from build123d import *

# Parameters (mm, degrees)
SKETCH1_W           = 304.8
SKETCH1_H           = 203.2
BOSS_EXTRUDE1_DEPTH = 228.6
SKETCH2_R           = 101.6
SKETCH2_R_2         = 76.2
BOSS_EXTRUDE2_DEPTH = 50.8
SKETCH3_R           = 38.1
CUT_EXTRUDE1_DEPTH  = 38.1
SKETCH4_W           = 203.2
SKETCH4_H           = 203.2
CUT_EXTRUDE2_DEPTH  = 190.5
SKETCH5_R           = 40.64
CUT_EXTRUDE3_DEPTH  = 304.8
FILLET1_R           = 101.6
CHAMFER1_SIZE       = 38.1


with BuildPart() as part:
    # Sketch1 → Boss-Extrude1 (new body)
    with BuildSketch(Plane(origin=(0, 0, 0), x_dir=(1, 0, 0), z_dir=(0, 1, 0))):
        Rectangle(SKETCH1_W, SKETCH1_H)
    extrude(amount=BOSS_EXTRUDE1_DEPTH)

    # Sketch2 → Boss-Extrude2 (add)
    with BuildSketch(Plane(origin=(0, 228.6, 0), x_dir=(1, 0, 0), z_dir=(0, 1, 0))):
        with Locations(Location((0, 0, 0), (0, 0, 270))):
            Circle(SKETCH2_R)
        with Locations(Location((0, 0, 0), (0, 0, 270))):
            Circle(SKETCH2_R_2, mode=Mode.SUBTRACT)
    extrude(amount=BOSS_EXTRUDE2_DEPTH)

    # Sketch3 → Cut-Extrude1 (cut)
    with BuildSketch(Plane(origin=(0, 228.6, 0), x_dir=(1, 0, 0), z_dir=(0, 1, 0))):
        with Locations(Location((0, 0, 0), (0, 0, 270))):
            Circle(SKETCH3_R)
    extrude(amount=-CUT_EXTRUDE1_DEPTH, mode=Mode.SUBTRACT)

    # Sketch4 → Cut-Extrude2 (cut)
    with BuildSketch(Plane.XZ):
        Rectangle(SKETCH4_W, SKETCH4_H)
    extrude(amount=-CUT_EXTRUDE2_DEPTH, mode=Mode.SUBTRACT)

    # Sketch5 → Cut-Extrude3 (cut)
    with BuildSketch(Plane(origin=(152.4, 0, 0), x_dir=(0, 0, -1), z_dir=(1, 0, 0))):
        with Locations((0, 101.6)):
            Circle(SKETCH5_R)
    extrude(amount=-CUT_EXTRUDE3_DEPTH, mode=Mode.SUBTRACT)

    # Fillet1
    fillet1_edges = [part.edges().sort_by_distance(p)[0] for p in [
        (127, 0, -101.6),
        (127, 0, 101.6),
        (-127, 0, -101.6),
        (-127, 0, 101.6),
    ]]
    fillet(fillet1_edges, radius=FILLET1_R - 0.0001)  # a hair under: the kernel refuses the full size

    # Chamfer1
    chamfer1_edges = [part.edges().sort_by_distance(p)[0] for p in [
        (0, 228.6, -38.1),
    ]]
    chamfer(chamfer1_edges, length=CHAMFER1_SIZE - 0.0001)  # a hair under: the kernel refuses the full size


solid = part.part
Model file for the job. Use its own axes, mm. A direction names the side the tool comes from. Coordinates: 2 decimals unless noted, no trailing zeros. Write each loop counter-clockwise with the first axis right and the second up, starting at its lowest first coordinate (ties: lowest second). Pieces come first, ordered by that corner, then holes. Notation, with made-up numbers: (-38, 8.5) - (-1, 8.5) arc R4 cw to (-1, 13.5) - close; hole circle Ø4 at (-22, 89.5). An arc over 180 degrees is marked (long way). Write each question's results on one line, items separated by ' | '. Start each with the question number.
1) Mould opens along X. For faces 6 (the face through (-126.644, 30.552, -72.628)), 7 (the face through (-39.521, 192.883, -8.776)), 8 (the face through (-152.4, 138, -21)) say: pulls with the +X half, pulls with the -X half, needs draft (parallel to the pull), parting line crosses it, or undercut.
2) Cut at D-D (y = 27). Write the cut outline in (x, z), then the cut area to 3 significant figures.
3) Cut at A-A (y = 109). Write the cut outline in (x, z).
4) Probe line 1 along Y through (x, z) = (-139, 0); line 2 along X through (y, z) = (61, 79); line 3 along Y through (x, z) = (71, 59). List the from-to ranges inside material, lowest first. Write a range as from..to.
5) Cut at C-C (z = 17). Count the separate pieces of the cut face and the enclosed holes in it, then the cut area to 3 significant figures.
6) Flat gauge pins, fed straight in: P1, Ø8, axis at x = -60, z = -27.5, coming from the +Y side; P2, Ø1, axis at x = -86, y = 248.5, coming from the -Z side; P3, Ø6, axis at x = 105.5, z = -67.5, coming from the +Y side. Where does each tip first touch, or does it go through?
7) 3-axis set-ups, long thin cutter, end or side, ignore diameter. For faces 1 (the face through (-101.6, 136, -24)), 2 (the face through (127.356, 30.552, 72.628)), 3 (the face through (-46.367, 253.644, -60.47)), 4 (the face through (-111, 228.6, -1)), 5 (the face through (109, 228.6, -1)): which of +Z, -Z, +X, -X, +Y, -Y reach the whole face in a straight line?
Returned:
1) face 6: needs draft | face 7: undercut | face 8: pulls with the -X half
2) outline: (-152.4, -68.97) - (-101.6, -68.97) - (-101.6, 68.97) - (-152.4, 68.97) - close; (101.6, -68.97) - (152.4, -68.97) - (152.4, 68.97) - (101.6, 68.97) - close | area: 14,000 mm^2
3) outline: (-152.4, -101.6) - (-101.6, -101.6) - (-101.6, -39.96) - (-152.4, -39.96) - close; (-152.4, 39.96) - (-101.6, 39.96) - (-101.6, 101.6) - (-152.4, 101.6) - close; (101.6, -101.6) - (152.4, -101.6) - (152.4, -39.96) - (101.6, -39.96) - close; (101.6, 39.96) - (152.4, 39.96) - (152.4, 101.6) - (101.6, 101.6) - close
4) line 1: 0..60.96, 142.24..228.6 | line 2: -152.4..-101.6, 101.6..152.4 | line 3: 190.5..279.4
5) separate pieces: 4 | enclosed holes: 0 | area: 21,800 mm^2
6) P1: y = 222.4 | P2: z = -54.88 | P3: y = 228.6
7) face 1: +Z, -Z, -Y | face 2: +Z, +X, -X, -Y | face 3: +Y | face 4: -X, +Y | face 5: +X, +Y
